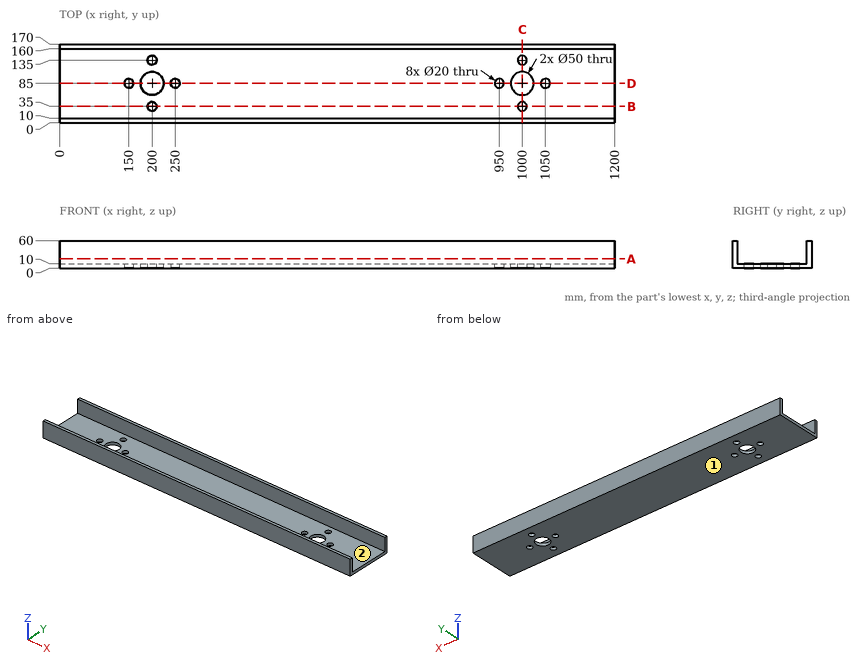
Design review of the part shown in the three views and the two pictorial views. Dimensions are in mm from the part's minimum x, y and z. Coordinates: 2 decimals unless noted, no trailing zeros. Loops run counter-clockwise (first coordinate to the right, second up) from the corner with the lowest first, then second, coordinate; pieces in that order, holes last. Notation, with made-up numbers: M -21,-28 L -17,-28 A21 cw -17,-18 Z; hole C 77,85.5 d11. An arc over 180 degrees is marked long. Put each result on its own line as item: value. Start each with the question number.
Q1. Wall thickness on line 1 (Y direction, x = 1143, z = 22); line 2 (Y direction, x = 150, z = 4.5); line 3 (Z direction, x = 168, y = 108): over which ranges is each line inside the solid? List them lowest first.
Q2. Add section C-C (x = 1000). Write out the cut boundary in (y, z).
Q3. Add section B-B (y = 35). Write out the cut boundary in (x, z), and give its area (3 significant figures).
Q4. Add section D-D (y = 85). Write out the cut boundary in (x, z), and give its area (3 significant figures).
Q5. Add section A-A (z = 20.5). Write out the cut boundary in (x, y).
Q6. The part is to be moulded in two halves that separate along Y. For the marked faces 1 and 2, say which applies: +Y half, -Y half, draft (parallel to the pull), parting line (faces both ways), or undercut.
Q7. Clearance check with flat-ended pins moving along their axes: pin 1 (12 mm diameter, centred on x = 950, y = 85, fed in from +Z); pin 2 (8 mm diameter, centred on x = 980, y = 134.5, fed in from +Z). State where each tip first meets the part, or that it passes through.
Answers:
1. line 1: y = 0 to 10, 160 to 170
1. line 2: y = 0 to 75, 95 to 170
1. line 3: z = 0 to 10
2. outline: M 0,0 L 25,0 L 25,10 L 10,10 L 10,60 L 0,60 Z; M 45,0 L 60,0 L 60,10 L 45,10 Z; M 110,0 L 125,0 L 125,10 L 110,10 Z; M 145,0 L 170,0 L 170,60 L 160,60 L 160,10 L 145,10 Z
3. outline: M 0,0 L 190,0 L 190,10 L 0,10 Z; M 210,0 L 990,0 L 990,10 L 210,10 Z; M 1010,0 L 1200,0 L 1200,10 L 1010,10 Z
3. area: 11,600 mm^2
4. outline: M 0,0 L 140,0 L 140,10 L 0,10 Z; M 160,0 L 175,0 L 175,10 L 160,10 Z; M 225,0 L 240,0 L 240,10 L 225,10 Z; M 260,0 L 940,0 L 940,10 L 260,10 Z; M 960,0 L 975,0 L 975,10 L 960,10 Z; M 1025,0 L 1040,0 L 1040,10 L 1025,10 Z; M 1060,0 L 1200,0 L 1200,10 L 1060,10 Z
4. area: 10,200 mm^2
5. outline: M 0,0 L 1200,0 L 1200,10 L 0,10 Z; M 0,160 L 1200,160 L 1200,170 L 0,170 Z
6. face 1: draft
6. face 2: undercut
7. pin 1: passes through
7. pin 2: stops at z = 10
